CAD build for the part. Positions are in the model's coordinates, mm. A direction names the side the tool comes from. Give positions to 0.01 mm unless a question says otherwise; leave off trailing zeros. Write each loop counter-clockwise with the first axis right and the second up, starting at its lowest first coordinate (ties: lowest second). Pieces come first, ordered by that corner, then holes. Notation, with made-up numbers: (49.5, 61.5) -> (72.5, 61.5) arc R17 ccw to (72.5, 71.5) -> close; hole circle Ø3 at (13.25, 30). An arc over 180 degrees is marked (long way). Use one line per item in the form item = value. Start each with the question number.
from build123d import *

# Parameters (mm, degrees)
F0_W     = 40
F0_H     = 40
F1_DEPTH = 3
F3_D     = 4
F4_R     = 5
F10_D    = 10


with BuildPart() as f1:
    # F0 (on Top) → F1 (new body)
    with BuildSketch(Plane.XY):
        with Locations((-20, 20)):
            Rectangle(F0_W, F0_H)
    extrude(amount=F1_DEPTH)

    # F3 (through all)
    with Locations(Plane.XY.offset(3)):
        with Locations((-34, 34)):
            Hole(F3_D / 2)

    # F4
    f4_edges = [f1.edges().sort_by_distance(p)[0] for p in [
        (-40, 40, 1.5),
    ]]
    fillet(f4_edges, radius=F4_R)

    # F5: F1 across face


with BuildPart() as f1_1:
    add(f1.part)
    add(f1.part.mirror(Plane(origin=(-20, 0, 1.5), x_dir=(1, 0, 0), z_dir=(0, -1, 0))))

    # F6: F1 across face


with BuildPart() as f1_2:
    add(f1_1.part)
    add(f1_1.part.mirror(Plane(origin=(0, 0, 1.5), x_dir=(0, 1, 0), z_dir=(1, 0, 0))))

    # F7 (on Front) → F8 (revolve)
    with BuildSketch(Plane.XZ):
        with BuildLine():
            Line((-40, 3), (0, 3))
            Line((0, 3), (0, 63))
            Line((0, 63), (-14, 63))
            Line((-14, 63), (-14, 58))
            Line((-14, 58), (-15, 58))
            ThreePointArc((-15, 58), (-16.5, 56.918861), (-18, 58))
            Line((-18, 58), (-19, 58))
            Line((-19, 58), (-19, 63))
            Line((-19, 63), (-24, 63))
            ThreePointArc((-24, 63), (-28.172502, 31.979334), (-40, 3))
        make_face()
    revolve(axis=Axis((0, 0, 33), (0, 0, 1)))

    # F10 (through all)
    with Locations(Plane.XY.offset(63)):
        with Locations((0, 0)):
            Hole(F10_D / 2)


solid = f1_2.part
1) Wall check: line 1 along Y through (x, z) = (-34, 1.1); line 2 along Z through (x, y) = (24, -35). Give the ranges that are in metal, low to high. Write a range as from..to.
2) Pin check, flat tips, straight feed: pin 1 (2 mm diameter, centred on x = -19.5, y = 28.5, fed in from +Z); pin 2 (4.5 mm diameter, centred on x = 34, y = -34, fed in from +Z); pin 3 (1.5 mm diameter, centred on x = 18, z = 25, fed in from +Y); pin 4 (1.5 mm diameter, centred on x = -24.5, y = -2.5, fed in from +Z). Stop position of each tip, or through.
3) Cut at B-B (z = 7.5). Give the cut face in (x, y).
4) Two-plate mould, pull along Y, no slides. Class faces 1 (the face through (-12.932, 5.362, 60.465)), 2 (the face through (39, -38, 2)), 3 (the face through (9, -1, 0)): released by +Y, released by -Y, zero draft, split by the parting line, or undercut.
5) Cut at A-A (z = 46). Give the cut face in (x, y), and give its area (3 significant figures).
6) 3-axis set-ups, long thin cutter, end or side, ignore diameter. For faces 4 (the face through (7, 17, 58)), 5 (the face through (30, -30, 3)), 6 (the face through (32, 30, 3)), 7 (the face through (-30, -30, 3)): which of +Z, -Z, +X, -X, +Y, -Y reach the whole face in a straight line?
Final values:
q1.line_1 = -40..-36, -32..32, 36..40
q1.line_2 = 0..3
q2.pin_1 = 16.22
q2.pin_2 = 3
q2.pin_3 = 24.94
q2.pin_4 = 63
q3.outline = circle Ø75.16 at (0, 0); hole circle Ø10 at (0, 0)
q4.face_1 = undercut
q4.face_2 = released by -Y
q4.face_3 = zero draft
q5.outline = circle Ø50.58 at (0, 0); hole circle Ø10 at (0, 0)
q5.area = 1,930 mm^2
q6.face_4 = +Z
q6.face_5 = +Z, +X, -Y
q6.face_6 = +Z, +X, +Y
q6.face_7 = +Z, -X, -Y
